Part model, mm, in its own coordinate system. A direction names the side the tool comes from. Give positions to 0.01 mm unless a question says otherwise; leave off trailing zeros. Write each loop counter-clockwise with the first axis right and the second up, starting at its lowest first coordinate (ties: lowest second). Pieces come first, ordered by that corner, then holes.
```python
from build123d import *

# Parameters (mm, degrees)
SKETCH_1_R           = 7
EXTRUDE_1_DEPTH      = 15
SKETCH_2_R           = 7
EXTRUDE_2_DEPTH      = 610
SKETCH_3_OUTSIDE_W   = 141.062
SKETCH_3_OUTSIDE_H   = 141.062
SKETCH_3_OUTSIDE_W_2 = 5
SKETCH_3_OUTSIDE_H_2 = 20
CUT_EXTRUDE_1_DEPTH  = 20
SKETCH_4_R           = 4
CUT_EXTRUDE_2_DEPTH  = 20


with BuildPart() as part:
    # 草图1 → 凸台-拉伸1 (new body)
    with BuildSketch(Plane(origin=(0, 0, 0), x_dir=(1, 0, 0), z_dir=(0, 1, 0))):
        Circle(SKETCH_1_R)
    extrude(amount=EXTRUDE_1_DEPTH)

    # 草图2 → 凸台-拉伸2 (add)
    with BuildSketch(Plane(origin=(0, 15, 0), x_dir=(1, 0, 0), z_dir=(0, 1, 0))):
        Circle(SKETCH_2_R)
    extrude(amount=EXTRUDE_2_DEPTH)

    # 草图3 outside → 切除-拉伸1 (cut)
    with BuildSketch(Plane(origin=(0, 625, 0), x_dir=(1, 0, 0), z_dir=(0, 1, 0))):
        Rectangle(SKETCH_3_OUTSIDE_W, SKETCH_3_OUTSIDE_H)
        Rectangle(SKETCH_3_OUTSIDE_W_2, SKETCH_3_OUTSIDE_H_2, mode=Mode.SUBTRACT)
    extrude(amount=-CUT_EXTRUDE_1_DEPTH, mode=Mode.SUBTRACT)

    # 草图4 → 切除-拉伸2 (cut)
    with BuildSketch(Plane.ZY.offset(2.5)):
        with Locations((0, 615)):
            Circle(SKETCH_4_R)
    extrude(amount=-CUT_EXTRUDE_2_DEPTH, mode=Mode.SUBTRACT)


solid = part.part
```
1) Saw through at B-B, the plane y = 526. Write the cut outline in (x, z), then the cut area to 3 significant figures.
Answers follow:
outline: circle Ø14 at (0, 0)
area: 154 mm2
2) Saw through at A-A, the plane z = 0. Write the cut outline in (x, y), then the cut area to 3 significant figures.
Answers follow:
outline: (-7, 0) - (7, 0) - (7, 605) - (2.5, 605) - (2.5, 611) - (-2.5, 611) - (-2.5, 605) - (-7, 605) - close; (-2.5, 619) - (2.5, 619) - (2.5, 625) - (-2.5, 625) - close
area: 8,530 mm2
3) 3-axis set-ups, long thin cutter, end or side, ignore diameter. For faces 1 (the face through (-2.5, 615.1, -4.3)), 2 (the face through (2.5, 615.1, -4.3)), 3 (the face through (0, 0, 0)): which of +Z, -Z, +X, -X, +Y, -Y reach the whole face in a straight line?
Answers follow:
face 1: +Z, -Z, -X, +Y
face 2: +Z, -Z, +X, +Y
face 3: +Z, -Z, +X, -X, -Y
4) Wall check: L1, parallel to Y at x = -1.35, z = 0; L2, parallel to Z at x = 0.55, y = 615; L3, parallel to X at y = 191.5, z = -0.5. Give the ranges that are in metal, low to high.
Answers follow:
L1: y = 0 to 611, 619 to 625
L2: z = -6.98 to -4, 4 to 6.98
L3: x = -6.98 to 6.98
5) Pin check, flat tips, straight feed: pin 1 Ø2 at (y, z) = (374.5, 4.5) entering from -X; pin 2 Ø1.3 at (x, z) = (-4.5, 1.5) entering from +Y; pin 3 Ø1.5 at (y, z) = (399.5, 5) entering from +X. Stop position of each tip, or through.
Answers follow:
pin 1: stops at x = -6.06
pin 2: stops at y = 605
pin 3: stops at x = 5.56
